```python
from build123d import *

# Parameters (mm, degrees)
SKETCH1_W           = 62.23
SKETCH1_H           = 25.9
BOSS_EXTRUDE1_DEPTH = 2
SKETCH2_R           = 1.524
SKETCH2_W           = 10.16
SKETCH2_H           = 8.12
CUT_EXTRUDE1_DEPTH  = 10


with BuildPart() as part:
    # Sketch1 → Boss-Extrude1 (new body)
    with BuildSketch(Plane(origin=(0, 0, 0), x_dir=(1, 0, 0), z_dir=(0, 1, 0))):
        with Locations((31.115, 12.95)):
            Rectangle(SKETCH1_W, SKETCH1_H)
    extrude(amount=BOSS_EXTRUDE1_DEPTH)

    # Sketch2 → Cut-Extrude1 (cut)
    with BuildSketch(Plane(origin=(0, 2, 0), x_dir=(1, 0, 0), z_dir=(0, 1, 0))):
        with Locations(Location((3.3, 22.6, 0), (0, 0, 270))):
            Circle(SKETCH2_R)
        with Locations(Location((3.3, 3.3, 0), (0, 0, 90))):
            Circle(SKETCH2_R)
        with Locations(Location((58.93, 3.3, 0), (0, 0, 270))):
            Circle(SKETCH2_R)
        with Locations(Location((58.93, 22.6, 0), (0, 0, 90))):
            Circle(SKETCH2_R)
        with Locations((38.735, 4.06)):
            Rectangle(SKETCH2_W, SKETCH2_H)
        with Locations((10.795, 4.06)):
            Rectangle(SKETCH2_W, SKETCH2_H)
        with Locations((51.435, 4.06)):
            Rectangle(SKETCH2_W, SKETCH2_H)
        with Locations((23.495, 4.06)):
            Rectangle(SKETCH2_W, SKETCH2_H)
    extrude(amount=-CUT_EXTRUDE1_DEPTH, mode=Mode.SUBTRACT)


solid = part.part
```
Read the model definition and answer for the solid it produces. Units are mm, in the model's axes. A direction names the side the tool comes from. Coordinates: 2 decimals unless noted, no trailing zeros. Write each loop counter-clockwise with the first axis right and the second up, starting at its lowest first coordinate (ties: lowest second). Pieces come first, ordered by that corner, then holes. Notation, with made-up numbers: (28.5, 68) -> (49.5, 68) arc R20 cw to (49.5, 98) -> close; hole circle Ø5 at (76.5, 38). An arc over 180 degrees is marked (long way). Return JSON: item names as keys, results as strings.
1. Determine the mould class of faces 1 (the face through (3, 1, 0)), 2 (the face through (31, 1, -25.9)), 3 (the face through (62.23, 1, -13)), 4 (the face through (2.7, 1, -21.2)) for opening direction Z: pulls with the +Z half, pulls with the -Z half, needs draft (parallel to the pull), parting line crosses it, or undercut.
Found:
{"face 1": "pulls with the +Z half", "face 2": "pulls with the -Z half", "face 3": "needs draft", "face 4": "undercut"}
2. A cutting plane is placed at A-A (y = 0.8). Determine the outline of the cut face in (x, z) (3 decimals).
Found:
{"outline": "(0, -25.9) -> (62.23, -25.9) -> (62.23, 0) -> (56.515, 0) -> (56.515, -8.12) -> (46.355, -8.12) -> (46.355, 0) -> (43.815, 0) -> (43.815, -8.12) -> (33.655, -8.12) -> (33.655, 0) -> (28.575, 0) -> (28.575, -8.12) -> (18.415, -8.12) -> (18.415, 0) -> (15.875, 0) -> (15.875, -8.12) -> (5.715, -8.12) -> (5.715, 0) -> (0, 0) -> close; hole circle Ø3.048 at (3.3, -22.6); hole circle Ø3.048 at (3.3, -3.3); hole circle Ø3.048 at (58.93, -22.6); hole circle Ø3.048 at (58.93, -3.3)"}
3. A cutting plane is placed at D-D (z = -22.6). Determine the outline of the cut face in (x, y).
Found:
{"outline": "(0, 0) -> (1.78, 0) -> (1.78, 2) -> (0, 2) -> close; (4.82, 0) -> (57.41, 0) -> (57.41, 2) -> (4.82, 2) -> close; (60.45, 0) -> (62.23, 0) -> (62.23, 2) -> (60.45, 2) -> close"}
4. A cutting plane is placed at C-C (z = -3.3). Determine the outline of the cut face in (x, y) (3 decimals), and give its area (3 significant figures).
Found:
{"outline": "(0, 0) -> (1.776, 0) -> (1.776, 2) -> (0, 2) -> close; (4.824, 0) -> (5.715, 0) -> (5.715, 2) -> (4.824, 2) -> close; (15.875, 0) -> (18.415, 0) -> (18.415, 2) -> (15.875, 2) -> close; (28.575, 0) -> (33.655, 0) -> (33.655, 2) -> (28.575, 2) -> close; (43.815, 0) -> (46.355, 0) -> (46.355, 2) -> (43.815, 2) -> close; (56.515, 0) -> (57.406, 0) -> (57.406, 2) -> (56.515, 2) -> close; (60.454, 0) -> (62.23, 0) -> (62.23, 2) -> (60.454, 2) -> close", "area": "31.0 mm2"}
5. This flat-tipped pin is pushed along its axis until it touches: P1, Ø1, axis at x = 49.5, y = 1, coming from the +Z side. Where does it stop, or does it pass through?
Found:
{"P1": "z = -8.12"}
6. Find the intervals of material crossed by line 1 along X through (y, z) = (0.7, -22.6); line 2 along Z through (x, y) = (59, 1.8); line 3 along X through (y, z) = (1, -7) (3 decimals), in increasing order. Write a range as from..to.
Found:
{"line 1": "0..1.78, 4.82..57.41, 60.45..62.23", "line 2": "-25.9..-24.12, -21.08..-4.82, -1.78..0", "line 3": "0..5.715, 15.875..18.415, 28.575..33.655, 43.815..46.355, 56.515..62.23"}
7. A tool of negligible diameter and unlimited length cuts with its end or side. For faces 5 (the face through (58.863, 1.014, -21.077)), 6 (the face through (39, 1, -8.12)), from which of +Z, -Z, +X, -X, +Y, -Y can it reach the whole face along a straight path? Write none if from no direction.
Found:
{"face 5": "+Y, -Y", "face 6": "+Z, +Y, -Y"}
8. A cutting plane is placed at B-B (x = 3.3). Determine the outline of the cut face in (y, z).
Found:
{"outline": "(0, -25.9) -> (2, -25.9) -> (2, -24.12) -> (0, -24.12) -> close; (0, -21.08) -> (2, -21.08) -> (2, -4.82) -> (0, -4.82) -> close; (0, -1.78) -> (2, -1.78) -> (2, 0) -> (0, 0) -> close"}
